Part model, mm, in its own coordinate system. Give positions to 0.01 mm unless a question says otherwise; leave off trailing zeros. Write each loop counter-clockwise with the first axis right and the second up, starting at its lowest first coordinate (ties: lowest second). Pieces come first, ordered by that corner, then holes. Notation, with made-up numbers: M 75,34 L 105,34 A31 ccw 105,60 Z; hole C 34,70 d10. An arc over 180 degrees is marked long. Use CSV: the item, a comma, the result in double quotes. Start each with the question number.
Item 1: Cut at C-C (x = 501.15). List the corners of the cut face in (y, z), then the cut area to 3 significant figures.
Item 2: Mould opens along Y. For faces 1 (the flat face through (420.666, 31.502, 0.681)), 2 (the flat face through (460, 22, 1.486)), 3 (the cylindrical face through (514.976, 45.462, 0.681)), 4 (the cylindrical face through (435.6, 16.64, 0.68)) say: released by +Y, released by -Y, zero draft, split by the parting line, or undercut.
Item 3: Pin check, flat tips, straight feed: pin 1 (3.5 mm diameter, centred on x = 424.95, y = 28.27, fed in from -Z); pin 2 (3 mm diameter, centred on x = 477.5, y = 2, fed in from +Z). Stop position of each tip, or through.
Item 4: Cut at B-B (x = 424.95). List the corners of the cut face in (y, z).
Item 5: Cut at A-A (z = 0.25). List the corners of the cut face in (x, y), then the cut area to 3 significant figures.
Item 6: Cut at D-D (x = 478.5). List the corners of the cut face in (y, z), then the cut area to 3 significant figures.
Item 7: Drill centre lines: line 1 (Y direction, x = 437.65, z = 0.6); line 2 (Y direction, x = 501.15, z = 0.45); line 3 (X direction, y = 28.5, z = 0.3). Where is each one in solid material? Low to high. Write a range as [from, to].
Autodesk Inventor part; units mm, degrees
ref_plane "Work Plane1" through (456.7, 53.6703, -0.1016) normal (0, 0, 1) x (0, 1, 0)
ref_plane "YZ Plane" through (0, 0, 0) normal (1, 0, 0) x (0, 1, 0)
ref_plane "XZ Plane" through (0, 0, 0) normal (0, 1, 0) x (-1, 0, 0)
ref_plane "Work Plane1" through (456.7, 53.6703, -0.1016) normal (0, 0, 1) x (0, 1, 0)
sketch "Sketch1" plane through (456.7, 53.6703, -0.1016) normal (0, 0, 1) x (0, 1, 0)
  circle A0 centre (-38.1, 19.05) radius 2.3114 construction
  circle A1 centre (-38.1, 31.75) radius 2.3114 construction
  circle A2 centre (-38.1, 31.75) radius 47.625 construction
  line L0 (-85.725, 31.75) -> (-85.725, -73.025) construction
  line L1 (-85.725, -73.025) -> (-69.85, -73.025) construction
  circle A3 centre (-39.624, -73.025) radius 30.226 construction
  line L2 (-63.4579, -9.6878) -> (-11.6843, -57.7145)
  line L3 (-6.35, -55.3867) -> (-6.35, 19.9759)
  line L4 (-70.4888, 2.6423) -> (-70.4888, 9.8614)
  arc A4 (-11.6843, -57.7145) -> (-6.35, -55.3867) centre (-9.525, -55.3867) ccw
  line L5 (-63.4579, -9.6878) -> (-69.473, -4.1079)
  line L6 (-70.4888, 2.6423) -> (-70.4888, -1.7802)
  arc A5 (-70.4888, -1.7802) -> (-69.473, -4.1079) centre (-67.3138, -1.7802) ccw
  circle A6 centre (-25.4, 31.75) radius 2.3114
  line L7 (-70.4888, -1.7802) -> (-70.4888, 22.2286)
  line L8 (-7.3657, 22.3036) -> (-37.3903, 50.1552)
  arc A7 (-6.35, 19.9759) -> (-7.3657, 22.3036) centre (-9.525, 19.9759) ccw
  line L9 (-69.466, 24.5628) -> (-41.7017, 50.1618)
  arc A8 (-37.3903, 50.1552) -> (-41.7017, 50.1618) centre (-39.5495, 47.8275) ccw
  arc A9 (-69.466, 24.5628) -> (-70.4888, 22.2286) centre (-67.3138, 22.2286) ccw
  circle A10 centre (-38.1, 19.05) radius 2.3114
  circle A11 centre (-25.4, 19.05) radius 2.3114
  circle A12 centre (-11.5316, -44.45) radius 2.3368
  circle A13 centre (-11.5316, -44.45) radius 2.1844 construction
  point P0 (-53.6703, 456.7)
  point P1 (-70.4888, -3.1657)
  point P2 (6.35, -48.768)
  point P3 (-6.35, 21.3614)
  point P4 (-19.05, 12.7)
  point P5 (-70.4888, 23.6198)
  dimension "d0" = 95.25
  dimension "d1" = 104.775
  dimension "d2" = 15.875
  dimension "d3" = 60.452
  dimension "d4" = 0
  dimension "d5" = 30.226
  dimension "d8" = 3.175
  dimension "d16" = 3.175
  dimension "d19" = 12.7
  dimension "d20" = 25.4
  dimension "d22" = 3.175
  dimension "d23" = 4.6736
  dimension "d26" = 63.5
  dimension "d29" = 0
extrude "Extrusion2" add sketch "Sketch1" along normal blind 1.5875 contours L5 A5 L6 L4 L7 A9 L9 A8 L8 A7 L3 A4 L2 | A11
properties part number "meow" material "Acetal Resin, White"
Worked answers:
1,outline,"M 27.69,-0.1 L 39.8,-0.1 L 39.8,1.49 L 27.69,1.49 Z; M 44.48,-0.1 L 47.32,-0.1 L 47.32,1.49 L 44.48,1.49 Z"
1,area,"23.7 mm^2"
2,face 1,"released by +Y"
2,face 2,"zero draft"
2,face 3,"split by the parting line"
2,face 4,"undercut"
3,pin 1,"passes through"
3,pin 2,"stops at z = 1.49"
4,outline,"M -8,-0.1 L 25.96,-0.1 L 25.96,1.49 L -8,1.49 Z; M 30.58,-0.1 L 36.12,-0.1 L 36.12,1.49 L 30.58,1.49 Z"
5,outline,"M 406.54,11.97 L 432.14,-15.8 A3.18 ccw 434.47,-16.82 L 458.48,-16.82 A3.17 ccw 460.81,-15.8 L 466.39,-9.79 L 514.41,41.99 A3.18 ccw 512.09,47.32 L 436.72,47.32 A3.18 ccw 434.4,46.3 L 406.54,16.28 A3.18 ccw Z; hole C 424.95,28.27 d4.62; hole C 437.65,15.57 d4.62; hole C 501.15,42.14 d4.67"
5,area,"4,440 mm^2"
6,outline,"M 3.27,-0.1 L 47.32,-0.1 L 47.32,1.49 L 3.27,1.49 Z"
6,area,"69.9 mm^2"
7,line 1,"y = [-16.82, 13.26], [17.88, 47.32]"
7,line 2,"y = [27.69, 39.8], [44.48, 47.32]"
7,line 3,"x = [417.88, 422.65], [427.25, 501.9]"
